Part model, mm, in its own coordinate system. A direction names the side the tool comes from. Coordinates: 2 decimals unless noted, no trailing zeros. Loops run counter-clockwise (first coordinate to the right, second up) from the corner with the lowest first, then second, coordinate; pieces in that order, holes last. Notation, with made-up numbers: (68.25, 80.5) -> (98.25, 80.5) arc R17 ccw to (98.25, 95.5) -> close; hole circle Ø5 at (55, -29.75). An arc over 180 degrees is marked (long way). Use one line per item in the form item = value. Start each with the question number.
(1) Band-saw the part on C-C on y = 0. Give the cut face in (x, z).
(2) Mould opens along X. For faces 3 (the flat face through (-16, 0, 109)), 4 (the flat face through (-19, 0, 109)), 5 (the cylindrical face through (-17.48, 3, 10.46)) say: +X half, -X half, draft (parallel to the pull), parting line (faces both ways), or undercut.
(3) Band-saw the part on A-A on z = 20. Give the cut face in (x, y), then the cut area to 3 significant figures.
(4) Band-saw the part on B-B on x = -4. Give the cut face in (y, z), then the cut area to 3 significant figures.
(5) Drill centre lines: L1, parallel to Y at x = 17.55, z = 210.68; L2, parallel to Y at x = 4, z = 194. Where is each one in solid material? Low to high. Write a range as [from, to].
(6) Pin check, flat tips, straight feed: P1, Ø6.5, axis at y = 10, z = 190.68, coming from the +X side; P2, Ø4, axis at y = 10, z = 190.68, coming from the -X side. Stop position of each tip, or through.
(7) Band-saw the part on D-D on z = 210.68. Give the cut face in (x, y), then the cut area to 3 significant figures.
(8) 3-axis set-ups, long thin cutter, end or side, ignore diameter. For faces 1 (the flat face through (0, 19, 109)), 2 (the flat face through (0, -16, 109)): which of +Z, -Z, +X, -X, +Y, -Y reach the whole face in a straight line?
```python
from build123d import *

# Parameters (mm, degrees)
SKETCH1_W               = 38
SKETCH1_H               = 38
SKETCH1_W_2             = 32
SKETCH1_H_2             = 32
BOSS_EXTRUDE1_DEPTH     = 220.68
SKETCH2_R               = 2.5
CUT_EXTRUDE1_DEPTH      = 1
CUT_EXTRUDE1_DEPTH_BACK = 39
SKETCH3_R               = 10
CUT_EXTRUDE2_DEPTH      = 39


with BuildPart() as part:
    # Sketch1 → Boss-Extrude1 (new body)
    with BuildSketch(Plane.XY):
        Rectangle(SKETCH1_W, SKETCH1_H)
        Rectangle(SKETCH1_W_2, SKETCH1_H_2, mode=Mode.SUBTRACT)
    extrude(amount=BOSS_EXTRUDE1_DEPTH)

    # Sketch2 → Cut-Extrude1 (cut, two sides)
    with BuildSketch(Plane.ZY.offset(19)) as cut_extrude1_sk:
        with Locations((190.68, -10)):
            Circle(SKETCH2_R)
        with Locations((210.68, -10)):
            Circle(SKETCH2_R)
        with Locations((190.68, 10)):
            Circle(SKETCH2_R)
        with Locations((210.68, 10)):
            Circle(SKETCH2_R)
    extrude(amount=CUT_EXTRUDE1_DEPTH, mode=Mode.SUBTRACT)
    extrude(cut_extrude1_sk.sketch, amount=-CUT_EXTRUDE1_DEPTH_BACK, mode=Mode.SUBTRACT)

    # Sketch3 → Cut-Extrude2 (cut, through all)
    with BuildSketch(Plane(origin=(19, 0, 0), x_dir=(0, 0, -1), z_dir=(1, 0, 0))):
        with Locations((-20, 0)):
            Circle(SKETCH3_R)
    extrude(amount=-CUT_EXTRUDE2_DEPTH, mode=Mode.SUBTRACT)


solid = part.part
```
A:
q1.outline = (-19, 0) -> (-16, 0) -> (-16, 10) -> (-19, 10) -> close; (-19, 30) -> (-16, 30) -> (-16, 220.68) -> (-19, 220.68) -> close; (16, 0) -> (19, 0) -> (19, 10) -> (16, 10) -> close; (16, 30) -> (19, 30) -> (19, 220.68) -> (16, 220.68) -> close
q2.face_3 = undercut
q2.face_4 = -X half
q2.face_5 = draft
q3.outline = (-19, -19) -> (19, -19) -> (19, -10) -> (16, -10) -> (16, -16) -> (-16, -16) -> (-16, -10) -> (-19, -10) -> close; (-19, 10) -> (-16, 10) -> (-16, 16) -> (16, 16) -> (16, 10) -> (19, 10) -> (19, 19) -> (-19, 19) -> close
q3.area = 300 mm²
q4.outline = (-19, 0) -> (-16, 0) -> (-16, 220.68) -> (-19, 220.68) -> close; (16, 0) -> (19, 0) -> (19, 220.68) -> (16, 220.68) -> close
q4.area = 1,320 mm²
q5.L1 = [-19, -12.5], [-7.5, 7.5], [12.5, 19]
q5.L2 = [-19, -16], [16, 19]
q6.P1 = 19
q6.P2 = through
q7.outline = (-19, -19) -> (19, -19) -> (19, -12.5) -> (16, -12.5) -> (16, -16) -> (-16, -16) -> (-16, -12.5) -> (-19, -12.5) -> close; (-19, -7.5) -> (-16, -7.5) -> (-16, 7.5) -> (-19, 7.5) -> close; (-19, 12.5) -> (-16, 12.5) -> (-16, 16) -> (16, 16) -> (16, 12.5) -> (19, 12.5) -> (19, 19) -> (-19, 19) -> close; (16, -7.5) -> (19, -7.5) -> (19, 7.5) -> (16, 7.5) -> close
q7.area = 360 mm²
q8.face_1 = +Z, -Z, +X, -X, +Y
q8.face_2 = +Z, -Z
